Geometry: final body of the model. Coordinates: model frame, mm. Coordinates: 2 decimals unless noted, no trailing zeros. Order: outer loops, then holes, each group sorted by start corner. A loop starts at its lowest first (then second) coordinate and runs counter-clockwise, first axis right, second up. Notation, with made-up numbers: (38, -21.5) -> (67, -21.5) arc R18 ccw to (67, 2.5) -> close; hole circle Ø8 at (8, 30). An arc over 180 degrees is marked (long way). Use one line per item in the form item = value.
```python
from build123d import *

# Parameters (mm, degrees)
SKETCH1_R           = 5.5
SKETCH1_R_2         = 3.25
BOSS_EXTRUDE1_DEPTH = 2


with BuildPart() as part:
    # Sketch1 → Boss-Extrude1 (new body)
    with BuildSketch(Plane.XY):
        with BuildLine():
            Line((68.948821818, 58.366235714), (29.948821818, 58.366235714))
            Line((29.948821818, 58.366235714), (29.948821818, 23.366235714))
            ThreePointArc((29.948821818, 23.366235714), (23.948821818, 17.366235714), (17.948821818, 23.366235714))
            Line((17.948821818, 23.366235714), (17.948821818, 58.366235714))
            Line((17.948821818, 58.366235714), (-180.051178182, 58.366235714))
            Line((-180.051178182, 58.366235714), (-180.051178182, 23.366235714))
            ThreePointArc((-180.051178182, 23.366235714), (-186.051178182, 17.366235714), (-192.051178182, 23.366235714))
            Line((-192.051178182, 23.366235714), (-192.051178182, 58.366235714))
            Line((-192.051178182, 58.366235714), (-231.051178182, 58.366235714))
            Line((-231.051178182, 58.366235714), (-231.051178182, -30.179856115))
            Line((-231.051178182, -30.179856115), (-261.051178182, -30.179856115))
            Line((-261.051178182, -30.179856115), (-261.051178182, -100.179856115))
            Line((-261.051178182, -100.179856115), (-231.051178182, -100.179856115))
            Line((-231.051178182, -100.179856115), (-231.051178182, -181.633764286))
            Line((-231.051178182, -181.633764286), (-192.051178182, -181.633764286))
            Line((-192.051178182, -181.633764286), (-192.051178182, -146.633764286))
            ThreePointArc((-192.051178182, -146.633764286), (-186.051178182, -140.633764286), (-180.051178182, -146.633764286))
            Line((-180.051178182, -146.633764286), (-180.051178182, -181.633764286))
            Line((-180.051178182, -181.633764286), (17.948821818, -181.633764286))
            Line((17.948821818, -181.633764286), (17.948821818, -146.633764286))
            ThreePointArc((17.948821818, -146.633764286), (23.948821818, -140.633764286), (29.948821818, -146.633764286))
            Line((29.948821818, -146.633764286), (29.948821818, -181.633764286))
            Line((29.948821818, -181.633764286), (68.948821818, -181.633764286))
            Line((68.948821818, -181.633764286), (68.948821818, -26.633764286))
            Line((68.948821818, -26.633764286), (68.948821818, 58.366235714))
        make_face()
        with Locations((-131.051178182, 13.486235714)):
            Circle(SKETCH1_R, mode=Mode.SUBTRACT)
        with Locations((53.948821818, -36.633764286)):
            Circle(SKETCH1_R_2, mode=Mode.SUBTRACT)
        with Locations((53.948821818, -86.633764286)):
            Circle(SKETCH1_R_2, mode=Mode.SUBTRACT)
        with Locations((-246.051178182, -65.179856115)):
            Circle(SKETCH1_R_2, mode=Mode.SUBTRACT)
        with Locations((-31.051178182, -136.753764286)):
            Circle(SKETCH1_R, mode=Mode.SUBTRACT)
        with Locations((-131.051178182, -136.753764286)):
            Circle(SKETCH1_R, mode=Mode.SUBTRACT)
        with Locations((-31.051178182, 13.486235714)):
            Circle(SKETCH1_R, mode=Mode.SUBTRACT)
    extrude(amount=BOSS_EXTRUDE1_DEPTH)


solid = part.part
```
1) Pull-direction query (X, two-part tool) for faces 1 (the cylindrical face through (56.95, -37.88, 0.99)), 2 (the flat face through (-98, -60, 0)); classes: released by +X, released by -X, zero draft, split by the parting line, or undercut.
Results found:
face_1 = undercut
face_2 = zero draft
2) Section D-D, the plane y = 3. Output: boundary loops of the cut face in (x, z).
Results found:
outline = (-231.05, 0) -> (68.95, 0) -> (68.95, 2) -> (-231.05, 2) -> close
3) Section C-C, the plane x = -238.5. Output: boundary loops of the cut face in (y, z).
Results found:
outline = (-100.18, 0) -> (-30.18, 0) -> (-30.18, 2) -> (-100.18, 2) -> close
4) Section B-B, the plane z = 1.05. Give the number of separate pieces and of enclosed holes in the cut face, and give its area (3 significant figures).
Results found:
separate_pieces = 1
enclosed_holes = 7
area = 71,700 mm2
5) Contact query for flat-ended pins moving along their axis: P1, Ø0.6, axis at y = 12, z = 1, coming from the -X side; P2, Ø10, axis at x = -31.05, y = 13.49, coming from the -Z side. Output: stop coordinate, or through.
Results found:
P1 = -231.05
P2 = through
6) Section A-A, the plane y = -162.5. Output: boundary loops of the cut face in (x, z).
Results found:
outline = (-231.05, 0) -> (-192.05, 0) -> (-192.05, 2) -> (-231.05, 2) -> close; (-180.05, 0) -> (17.95, 0) -> (17.95, 2) -> (-180.05, 2) -> close; (29.95, 0) -> (68.95, 0) -> (68.95, 2) -> (29.95, 2) -> close
7) Material intervals for probe 1 along X at (y, z) = (36, 1.15); probe 2 along X at (y, z) = (22, 0.45); probe 3 along Y at (x, z) = (-27.5, 1), sorted ascending. Write a range as from..to.
Results found:
probe_1 = -231.05..-192.05, -180.05..17.95, 29.95..68.95
probe_2 = -231.05..-191.89, -180.21..18.11, 29.79..68.95
probe_3 = -181.63..-140.95, -132.55..9.29, 17.69..58.37
